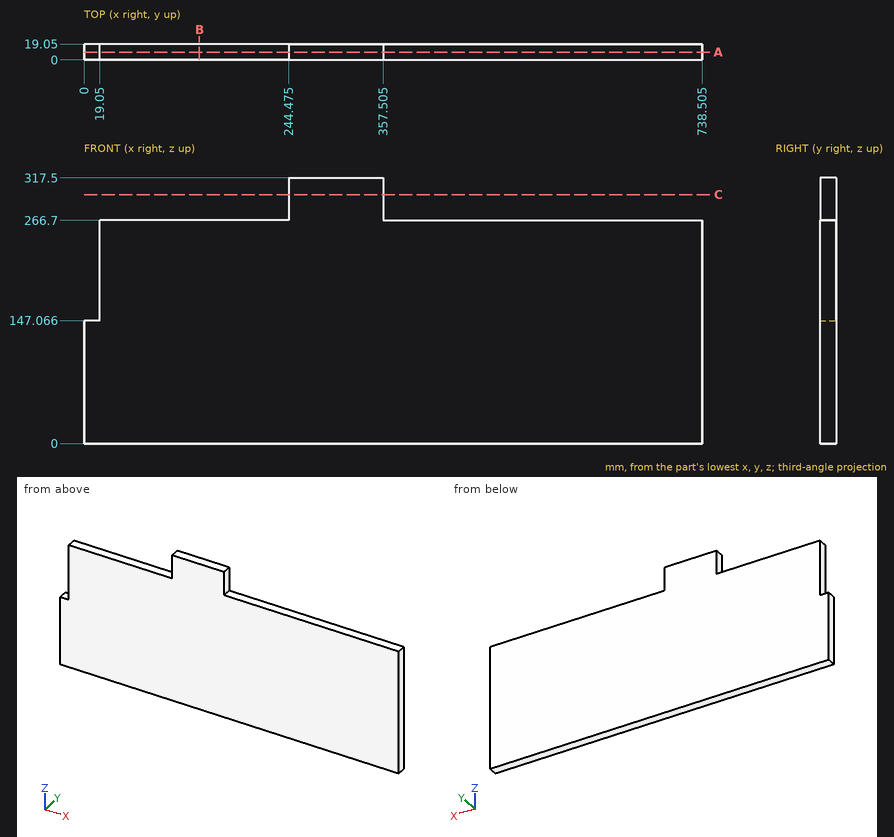
Part print with two shaded views. Sizes in mm from the minimum x, y, z corner. Coordinates: 2 decimals unless noted, no trailing zeros. Write each loop counter-clockwise with the first axis right and the second up, starting at its lowest first coordinate (ties: lowest second). Pieces come first, ordered by that corner, then holes.
1. Band-saw the part on B-B, the plane x = 138. Give the cut face in (y, z).
Answer block:
outline: (0, 0) - (19.05, 0) - (19.05, 266.7) - (0, 266.7) - close
2. Band-saw the part on A-A, the plane y = 9.25. Give the cut face in (x, z) (3 decimals), and give its area (3 significant figures).
Answer block:
outline: (0, 0) - (738.505, 0) - (738.505, 266.7) - (357.505, 266.7) - (357.505, 317.5) - (244.475, 317.5) - (244.475, 266.7) - (19.05, 266.7) - (19.05, 147.066) - (0, 147.066) - close
area: 200,000 mm2
3. Band-saw the part on C-C, the plane z = 297.5. Give the cut face in (x, y) (3 decimals), and give its area (3 significant figures).
Answer block:
outline: (244.475, 0) - (357.505, 0) - (357.505, 19.05) - (244.475, 19.05) - close
area: 2,150 mm2
4. Drop flat-ended pins along their axis: pin 1 (8 mm diameter, centred on x = 430.5, y = 13, fed in from +Z); pin 2 (2 mm diameter, centred on y = 3.5, z = 47.5, fed in from -X); pin 3 (9.5 mm diameter, centred on y = 8.5, z = 300.5, fed in from -X) (3 decimals); pin 4 (5.5 mm diameter, centred on y = 9, z = 211.5, fed in from -X). Give the stop position or say it passes through.
Answer block:
pin 1: stops at z = 266.7
pin 2: stops at x = 0
pin 3: stops at x = 244.475
pin 4: stops at x = 19.05
5. Drill centre lines: probe 1 along Z at (x, y) = (225, 1.5); probe 2 along X at (y, z) = (13.5, 169.5) (3 decimals); probe 3 along X at (y, z) = (13.25, 300) (3 decimals). Where is each one in solid material? Low to high.
Answer block:
probe 1: z = 0 to 266.7
probe 2: x = 19.05 to 738.505
probe 3: x = 244.475 to 357.505
